Source: CAD feature listing. Evaluate the final solid. Frame: model axes, mm. Face numbers are marked on the shaded views. A direction names the side the tool comes from. Give positions to 0.01 mm unless a question says otherwise; leave off trailing zeros. Loops run counter-clockwise (first coordinate to the right, second up) from the corner with the lowest first, then second, coordinate; pieces in that order, holes last. Notation, with made-up numbers: (47, -25) - (52, -25) arc R20 cw to (52, -7) - close; hole circle Ø3 at (45, 77.5). An arc over 180 degrees is marked (long way). Put each result on its own line as item: value.
Autodesk Inventor part; units mm, degrees
ref_plane "YZ Plane" through (0, 0, 0) normal (1, 0, 0) x (0, 1, 0)
ref_plane "XZ Plane" through (0, 0, 0) normal (0, 1, 0) x (-1, 0, 0)
ref_plane "XY Plane" through (0, 0, 0) normal (0, 0, 1) x (1, 0, 0)
sketch "Sketch1" plane through (0, 0, 0) normal (0, 1, 0) x (-1, 0, 0)
  spline S0 degree 3 poles (19.0088, -20.3781) (18.4587, -20.3781) (18.0142, -19.9334) (18.0142, -19.3832) (18.0142, -18.833) (18.4587, -18.3883) (19.0088, -18.3883) (19.5594, -18.3883) (20.0038, -18.833) (20.0038, -19.3832) (20.0038, -19.9334) (19.5594, -20.3781) (19.0088, -20.3781) knots 0 0 0 0 1 1 1 2 2 2 3 3 3 4 4 4 4
  line L0 (19.0088, -20.3781) -> (18.4587, -20.3781) construction
  line L1 (18.4587, -20.3781) -> (18.0142, -19.9334) construction
  line L2 (18.0142, -19.9334) -> (18.0142, -19.3832) construction
  line L3 (18.0142, -19.3832) -> (18.0142, -18.833) construction
  line L4 (18.0142, -18.833) -> (18.4587, -18.3883) construction
  line L5 (18.4587, -18.3883) -> (19.0088, -18.3883) construction
  line L6 (19.0088, -18.3883) -> (19.5594, -18.3883) construction
  line L7 (19.5594, -18.3883) -> (20.0038, -18.833) construction
  line L8 (20.0038, -18.833) -> (20.0038, -19.3832) construction
  line L9 (20.0038, -19.3832) -> (20.0038, -19.9334) construction
  line L10 (20.0038, -19.9334) -> (19.5594, -20.3781) construction
  line L11 (19.5594, -20.3781) -> (19.0088, -20.3781) construction
  spline S1 degree 3 poles (19.0088, -20.3781) (18.4587, -20.3781) (18.0142, -19.9334) (18.0142, -19.3832) (18.0142, -18.833) (18.4587, -18.3883) (19.0088, -18.3883) (19.5594, -18.3883) (20.0038, -18.833) (20.0038, -19.3832) (20.0038, -19.9334) (19.5594, -20.3781) (19.0088, -20.3781) knots 0 0 0 0 1 1 1 2 2 2 3 3 3 4 4 4 4
  line L12 (19.0088, -20.3781) -> (18.4587, -20.3781) construction
  line L13 (18.4587, -20.3781) -> (18.0142, -19.9334) construction
  line L14 (18.0142, -19.9334) -> (18.0142, -19.3832) construction
  line L15 (18.0142, -19.3832) -> (18.0142, -18.833) construction
  line L16 (18.0142, -18.833) -> (18.4587, -18.3883) construction
  line L17 (18.4587, -18.3883) -> (19.0088, -18.3883) construction
  line L18 (19.0088, -18.3883) -> (19.5594, -18.3883) construction
  line L19 (19.5594, -18.3883) -> (20.0038, -18.833) construction
  line L20 (20.0038, -18.833) -> (20.0038, -19.3832) construction
  line L21 (20.0038, -19.3832) -> (20.0038, -19.9334) construction
  line L22 (20.0038, -19.9334) -> (19.5594, -20.3781) construction
  line L23 (19.5594, -20.3781) -> (19.0088, -20.3781) construction
  spline S2 degree 3 poles (19.0088, -5.1804) (18.4587, -5.1804) (18.0142, -4.7359) (18.0142, -4.1855) (18.0142, -3.6352) (18.4587, -3.1907) (19.0088, -3.1907) (19.5594, -3.1907) (20.0038, -3.6352) (20.0038, -4.1855) (20.0038, -4.7359) (19.5594, -5.1804) (19.0088, -5.1804) knots 0 0 0 0 1 1 1 2 2 2 3 3 3 4 4 4 4
  line L24 (19.0088, -5.1804) -> (18.4587, -5.1804) construction
  line L25 (18.4587, -5.1804) -> (18.0142, -4.7359) construction
  line L26 (18.0142, -4.7359) -> (18.0142, -4.1855) construction
  line L27 (18.0142, -4.1855) -> (18.0142, -3.6352) construction
  line L28 (18.0142, -3.6352) -> (18.4587, -3.1907) construction
  line L29 (18.4587, -3.1907) -> (19.0088, -3.1907) construction
  line L30 (19.0088, -3.1907) -> (19.5594, -3.1907) construction
  line L31 (19.5594, -3.1907) -> (20.0038, -3.6352) construction
  line L32 (20.0038, -3.6352) -> (20.0038, -4.1855) construction
  line L33 (20.0038, -4.1855) -> (20.0038, -4.7359) construction
  line L34 (20.0038, -4.7359) -> (19.5594, -5.1804) construction
  line L35 (19.5594, -5.1804) -> (19.0088, -5.1804) construction
  spline S3 degree 3 poles (19.0088, -5.1804) (18.4587, -5.1804) (18.0142, -4.7359) (18.0142, -4.1855) (18.0142, -3.6352) (18.4587, -3.1907) (19.0088, -3.1907) (19.5594, -3.1907) (20.0038, -3.6352) (20.0038, -4.1855) (20.0038, -4.7359) (19.5594, -5.1804) (19.0088, -5.1804) knots 0 0 0 0 1 1 1 2 2 2 3 3 3 4 4 4 4
  line L36 (19.0088, -5.1804) -> (18.4587, -5.1804) construction
  line L37 (18.4587, -5.1804) -> (18.0142, -4.7359) construction
  line L38 (18.0142, -4.7359) -> (18.0142, -4.1855) construction
  line L39 (18.0142, -4.1855) -> (18.0142, -3.6352) construction
  line L40 (18.0142, -3.6352) -> (18.4587, -3.1907) construction
  line L41 (18.4587, -3.1907) -> (19.0088, -3.1907) construction
  line L42 (19.0088, -3.1907) -> (19.5594, -3.1907) construction
  line L43 (19.5594, -3.1907) -> (20.0038, -3.6352) construction
  line L44 (20.0038, -3.6352) -> (20.0038, -4.1855) construction
  line L45 (20.0038, -4.1855) -> (20.0038, -4.7359) construction
  line L46 (20.0038, -4.7359) -> (19.5594, -5.1804) construction
  line L47 (19.5594, -5.1804) -> (19.0088, -5.1804) construction
  line L48 (19.0302, -21.9233) -> (19.4746, -21.9019)
  spline S4 degree 3 poles (19.4746, -21.9019) (20.5647, -21.6366) (21.3157, -20.9538) (21.5279, -19.8276) knots 1 1 1 1 2 2 2 2
  line L49 (19.4746, -21.9019) -> (20.5647, -21.6366) construction
  line L50 (20.5647, -21.6366) -> (21.3157, -20.9538) construction
  line L51 (21.3157, -20.9538) -> (21.5279, -19.8276) construction
  line L52 (21.5279, -19.8276) -> (21.5703, -19.4042)
  line L53 (21.5703, -19.4042) -> (21.5703, -4.1855)
  line L54 (21.5703, -4.1855) -> (21.5279, -3.7411)
  spline S5 degree 3 poles (21.5279, -3.7411) (21.3143, -2.6778) (20.5474, -1.8728) (19.4746, -1.6878) knots 5 5 5 5 6 6 6 6
  line L55 (21.5279, -3.7411) -> (21.3143, -2.6778) construction
  line L56 (21.3143, -2.6778) -> (20.5474, -1.8728) construction
  line L57 (20.5474, -1.8728) -> (19.4746, -1.6878) construction
  line L58 (19.4746, -1.6878) -> (19.0302, -1.6456)
  line L59 (19.0302, -1.6456) -> (3.8115, -1.6456)
  line L60 (3.8115, -1.6456) -> (3.3881, -1.6878)
  spline S6 degree 3 poles (3.3881, -1.6878) (2.3177, -1.8298) (1.536, -2.7195) (1.3138, -3.7411) knots 9 9 9 9 10 10 10 10
  line L61 (3.3881, -1.6878) -> (2.3177, -1.8298) construction
  line L62 (2.3177, -1.8298) -> (1.536, -2.7195) construction
  line L63 (1.536, -2.7195) -> (1.3138, -3.7411) construction
  line L64 (1.3138, -3.7411) -> (1.2924, -4.1855)
  line L65 (1.2924, -4.1855) -> (1.2924, -19.4042)
  line L66 (1.2924, -19.4042) -> (1.3138, -19.8276)
  spline S7 degree 3 poles (1.3138, -19.8276) (1.5308, -20.908) (2.308, -21.6852) (3.3881, -21.9019) knots 13 13 13 13 14 14 14 14
  line L67 (1.3138, -19.8276) -> (1.5308, -20.908) construction
  line L68 (1.5308, -20.908) -> (2.308, -21.6852) construction
  line L69 (2.308, -21.6852) -> (3.3881, -21.9019) construction
  line L70 (3.3881, -21.9019) -> (3.8115, -21.9233)
  line L71 (3.8115, -21.9233) -> (19.0302, -21.9233)
  point P0 (0, 0)
sketch "Sketch2" plane through (0, 0, 0) normal (0, 1, 0) x (-1, 0, 0)
  line L0 (19.5198, -21.9426) -> (6.2891, -21.9426)
  line L1 (4.2891, -19.9426) -> (4.2891, -3.657)
  line L2 (6.2891, -1.657) -> (19.5198, -1.657)
  line L3 (21.5198, -3.657) -> (21.5198, -19.9426)
  arc A0 (21.5198, -3.657) -> (19.5198, -1.657) centre (19.5198, -3.657) ccw
  arc A1 (19.5198, -21.9426) -> (21.5198, -19.9426) centre (19.5198, -19.9426) ccw
  arc A2 (4.2891, -19.9426) -> (6.2891, -21.9426) centre (6.2891, -19.9426) ccw
  arc A3 (6.2891, -1.657) -> (4.2891, -3.657) centre (6.2891, -3.657) ccw
  circle A4 centre (19.1022, -4.1405) radius 1.5
  circle A5 centre (19.1022, -19.4152) radius 1.5
  line L4 (21.5198, -5.825) -> (9.7891, -5.825)
  line L5 (9.7891, -5.825) -> (9.7891, -17.9152)
  line L6 (9.7891, -17.9152) -> (21.5198, -17.9152)
  point P0 (0, 0)
  dimension "d0" = 2
  dimension "d1" = 3
  dimension "d2" = 3
extrude "Extrusion1" add sketch "Sketch2" along normal blind 9 contours L0 A2 L1 A3 L2 A0 L3 L4 L5 L6 A1
properties part number "thermo-model"
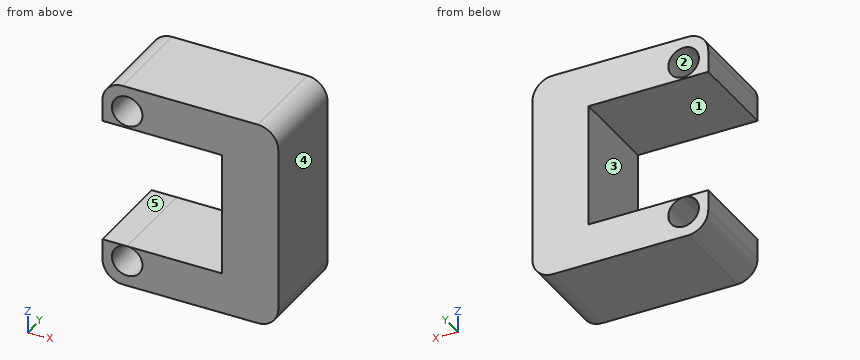
1) Section query D-D, the plane z = -17.25. Output: boundary loops of the cut face in (x, y), plus the area to 3 significant figures.
Check result:
outline: (-9.79, 0) - (-4.29, 0) - (-4.29, 9) - (-9.79, 9) - close
area: 49.5 mm²
2) Section query B-B, the plane z = -5. Output: boundary loops of the cut face in (x, y), plus the area to 3 significant figures.
Check result:
outline: (-21.52, 0) - (-20.33, 0) - (-20.33, 9) - (-21.52, 9) - close; (-17.87, 0) - (-4.29, 0) - (-4.29, 9) - (-17.87, 9) - close
area: 133 mm²
3) Section query A-A, the plane x = -14.25. Output: boundary loops of the cut face in (y, z) (3 decimals).
Check result:
outline: (0, -21.943) - (9, -21.943) - (9, -17.915) - (0, -17.915) - close; (0, -5.825) - (9, -5.825) - (9, -1.657) - (0, -1.657) - close
4) Mould query, pull axis X, two halves, no side actions, for the marked faces 1, 2 and 3. Classes: pulls with the +X half, pulls with the -X half, needs draft (parallel to the pull), parting line crosses it, or undercut.
Check result:
face 1: needs draft
face 2: undercut
face 3: pulls with the -X half
5) Access query for the marked faces 4 and 5. Directions: +Z, -Z, +X, -X, +Y, -Y. A direction counts if a zero-diameter tool reaches every point of the face in a straight line with its end or side. Return the directions, or none.
Check result:
face 4: +Z, -Z, +X, +Y, -Y
face 5: -X, +Y, -Y
6) Material intervals for line 1 along Z through (x, y) = (-16.5, 2.5) (3 decimals); line 2 along X through (y, z) = (6.25, -6.5); line 3 along X through (y, z) = (0.5, -18.75), sorted ascending. Write a range as [from, to].
Check result:
line 1: [-21.943, -17.915], [-5.825, -1.657]
line 2: [-9.79, -4.29]
line 3: [-21.52, -20.45], [-17.76, -4.29]
7) Pin query (flat end, axial travel): P1, Ø0.7, axis at x = -20.5, y = 6.5, coming from the +Z side. Return the tip coordinate at first contact, or that it passes through.
Check result:
P1: z = -1.76
